Check sheet for the drawn part. Datum: minimum x, y, z corner. Units: mm. A direction names the side the tool comes from. Coordinates: 2 decimals unless noted, no trailing zeros. Write each loop counter-clockwise with the first axis right and the second up, starting at its lowest first coordinate (ties: lowest second). Pieces come first, ordered by that corner, then holes. Notation, with made-up numbers: (-33.5, 51) -> (8.5, 51) arc R24 cw to (8.5, 70) -> close; hole circle Ø9 at (32, 15.5). An arc over 180 degrees is marked (long way). Write item = value, one per line. Start each with the question number.
(1) Mould release check, pull along Y, two halves, no side actions. Record for the marked faces 4, 5 and 6: released by +Y, released by -Y, zero draft, split by the parting line, or undercut.
(2) Material ranges on probe 1 along Y at (x, z) = (3, 1.5); probe 2 along Y at (x, z) = (25, 4); probe 3 along Z at (x, y) = (23.5, 13.25), recorded low to high. Write a range as [from, to].
(3) Section check D-D (x = 21). Record the cut outline in (y, z), plus the area to 3 significant figures.
(4) Section check C-C (y = 7). Record the cut outline in (x, z), plus the area to 3 significant figures.
(5) Set-up check for the marked faces 1, 2 and 3: record each of +Z, -Z, +X, -X, +Y, -Y from which the full face is reachable in a straight line by a thin tool's end or side.
(6) Section check B-B (z = 8.75). Record the cut outline in (x, y).
(7) Gauge pin test, flat end, axial feed: pin 1 Ø6 at (x, y) = (25, 10) entering from +Z. Record the tip position at first contact, or that the pin passes through.
(8) Section check A-A (x = 25). Record the cut outline in (y, z), plus the area to 3 significant figures.
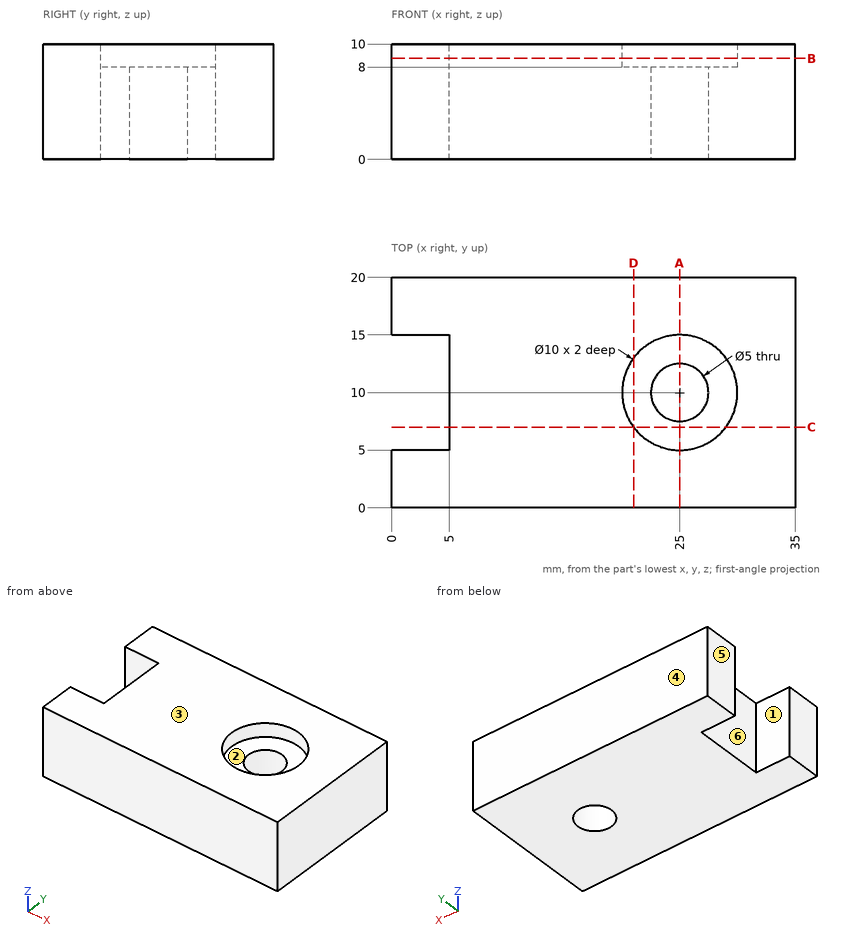
Response:
q1.face_4 = released by +Y
q1.face_5 = zero draft
q1.face_6 = undercut
q2.probe_1 = [0, 5], [15, 20]
q2.probe_2 = [0, 7.5], [12.5, 20]
q2.probe_3 = [0, 8]
q3.outline = (0, 0) -> (20, 0) -> (20, 10) -> (13, 10) -> (13, 8) -> (7, 8) -> (7, 10) -> (0, 10) -> close
q3.area = 188 mm2
q4.outline = (5, 0) -> (35, 0) -> (35, 10) -> (29, 10) -> (29, 8) -> (21, 8) -> (21, 10) -> (5, 10) -> close
q4.area = 284 mm2
q5.face_1 = +Z, -Z, -X
q5.face_2 = +Z
q5.face_3 = +Z, +X, -X, +Y, -Y
q6.outline = (0, 0) -> (35, 0) -> (35, 20) -> (0, 20) -> (0, 15) -> (5, 15) -> (5, 5) -> (0, 5) -> close; hole circle Ø10 at (25, 10)
q7.pin_1 = 8
q8.outline = (0, 0) -> (7.5, 0) -> (7.5, 8) -> (5, 8) -> (5, 10) -> (0, 10) -> close; (12.5, 0) -> (20, 0) -> (20, 10) -> (15, 10) -> (15, 8) -> (12.5, 8) -> close
q8.area = 140 mm2
